from build123d import *

# Parameters (mm, degrees)
SKETCH1_R           = 2
SKETCH1_R_2         = 2.5
BOSS_EXTRUDE1_DEPTH = 5


with BuildPart() as part:
    # Sketch1 → Boss-Extrude1 (new body)
    with BuildSketch(Plane(origin=(0, 0, 701.677889561), x_dir=(-1, 0, 0), z_dir=(0, 0, -1))):
        with BuildLine():
            Line((-99.719780497, 143.525710146), (-99.719780497, 111.833409744))
            ThreePointArc((-99.719780497, 111.833409744), (-99.09450302, 109.686028108), (-97.41415655, 108.210001157))
            ThreePointArc((-97.41415655, 108.210001157), (-102.311705141, 85.341210472), (-107.91415655, 108.047599613))
            ThreePointArc((-107.91415655, 108.047599613), (-106.312252376, 109.521939482), (-105.719780497, 111.616874352))
            Line((-105.719780497, 111.616874352), (-105.719780497, 143.525710146))
            ThreePointArc((-105.719780497, 143.525710146), (-106.891353372, 146.354137271), (-109.719780497, 147.525710146))
            Line((-109.719780497, 147.525710146), (-150.816081745, 147.525710146))
            ThreePointArc((-150.816081745, 147.525710146), (-152.230295307, 146.939923708), (-152.816081745, 145.525710146))
            Line((-152.816081745, 145.525710146), (-152.816081745, 49.525710146))
            ThreePointArc((-152.816081745, 49.525710146), (-152.230295307, 48.111496583), (-150.816081745, 47.525710146))
            Line((-150.816081745, 47.525710146), (-54.816081745, 47.525710146))
            ThreePointArc((-54.816081745, 47.525710146), (-53.401868182, 48.111496583), (-52.816081745, 49.525710146))
            Line((-52.816081745, 49.525710146), (-52.816081745, 145.525710146))
            ThreePointArc((-52.816081745, 145.525710146), (-53.401868182, 146.939923708), (-54.816081745, 147.525710146))
            Line((-54.816081745, 147.525710146), (-95.719780497, 147.525710146))
            ThreePointArc((-95.719780497, 147.525710146), (-98.548207622, 146.354137271), (-99.719780497, 143.525710146))
        make_face()
        with Locations(Location((-87.123479249, 81.839775395, 0), (0, 0, 180))):
            Circle(SKETCH1_R, mode=Mode.SUBTRACT)
        with Locations(Location((-118.123479249, 81.839775395, 0), (0, 0, 180))):
            Circle(SKETCH1_R, mode=Mode.SUBTRACT)
        with Locations(Location((-87.123479249, 112.839775395, 0), (0, 0, 180))):
            Circle(SKETCH1_R, mode=Mode.SUBTRACT)
        with Locations(Location((-118.123479249, 112.839775395, 0), (0, 0, 180))):
            Circle(SKETCH1_R, mode=Mode.SUBTRACT)
        with Locations(Location((-102.816081745, 57.525710146, 0), (0, 0, 180))):
            Circle(SKETCH1_R_2, mode=Mode.SUBTRACT)
        with Locations(Location((-62.816081745, 137.525710146, 0), (0, 0, 180))):
            Circle(SKETCH1_R_2, mode=Mode.SUBTRACT)
        with Locations(Location((-142.816081745, 137.525710146, 0), (0, 0, 180))):
            Circle(SKETCH1_R_2, mode=Mode.SUBTRACT)
        with Locations(Location((-64.816081745, 97.525710146, 0), (0, 0, 180))):
            Circle(SKETCH1_R, mode=Mode.SUBTRACT)
        with Locations(Location((-140.816081745, 97.525710146, 0), (0, 0, 180))):
            Circle(SKETCH1_R, mode=Mode.SUBTRACT)
    extrude(amount=-BOSS_EXTRUDE1_DEPTH)


solid = part.part
Design review of the part built by this model. Coordinates are the model's own, in mm. A direction names the side the tool comes from. Give positions to 0.01 mm unless a question says otherwise; leave off trailing zeros. Loops run counter-clockwise (first coordinate to the right, second up) from the corner with the lowest first, then second, coordinate; pieces in that order, holes last. Notation, with made-up numbers: M -15,20.25 L 29,20.25 A31 cw 29,50.25 Z; hole C 57,12.25 d3. An arc over 180 degrees is marked long. One line per question, with ' | ' between items. Start each with the question number.
1. Insertion check: P1, Ø21.5, axis at x = 102.5, y = 97.34, coming from the -Z side; P2, Ø6, axis at x = 142.82, y = 137.53, coming from the +Z side. Each pin has a flat end and moves straight along its axis. Give the tip position at first contact, or say it passes through.
2. To check wall thickness, follow L1, parallel to X at y = 132, z = 703.35; L2, parallel to X at y = 139, z = 703.7; L3, parallel to Y at x = 119, z = 702.5. State the ranges of each line that lie inside material, in increasing order.
3. The part is to be moulded in two halves that separate along X. For faces 4 (the face through (99.11, 109.71, 704.14)), 5 (the face through (152.816, 98, 704)), 6 (the face through (75, 147.526, 704)), say which applies: released by +X, released by -X, zero draft, split by the parting line, or undercut.
4. Add section C-C (z = 704.55). Give the number of separate pieces and of enclosed holes in the cut face, plus the area to 3 significant figures.
5. Add section A-A (y = 125). Write out the cut boundary in (x, z).
6. For faces 1 (the face through (130, 147.526, 704)), 2 (the face through (106.329, 109.496, 704.143)), 3 (the face through (105.72, 127, 704)), list the 3-axis set-ups (+Z, -Z, +X, -X, +Y, -Y) from which the entire face can be reached by the end or side of a thin tool; tool diameter is ignored.
7. Add section B-B (x = 93). Write out the cut boundary in (y, z).
Worked out:
1) P1: passes through | P2: stops at z = 706.68
2) L1: x = 52.82 to 99.72, 105.72 to 152.82 | L2: x = 52.82 to 60.8, 64.84 to 99.72, 105.72 to 140.8, 144.84 to 152.82 | L3: y = 47.53 to 80.04, 83.64 to 111.04, 114.64 to 147.53
3) face 4: undercut | face 5: released by +X | face 6: zero draft
4) separate pieces: 1 | enclosed holes: 9 | area: 9,170 mm²
5) outline: M 52.82,701.68 L 99.72,701.68 L 99.72,706.68 L 52.82,706.68 Z; M 105.72,701.68 L 152.82,701.68 L 152.82,706.68 L 105.72,706.68 Z
6) face 1: +Z, -Z, +X, -X, +Y | face 2: +Z, -Z | face 3: +Z, -Z, +Y
7) outline: M 47.53,701.68 L 90,701.68 L 90,706.68 L 47.53,706.68 Z; M 104.67,701.68 L 147.53,701.68 L 147.53,706.68 L 104.67,706.68 Z
